from build123d import *

# Parameters (mm, degrees)
SKETCH1_R           = 3.2639
BOSS_EXTRUDE1_DEPTH = 1.5875
SKETCH2_R           = 12.7
CUT_EXTRUDE1_DEPTH  = 27.658658303


with BuildPart() as part:
    # Sketch1 → Boss-Extrude1 (new body)
    with BuildSketch(Plane(origin=(0, 0, 0), x_dir=(1, 0, 0), z_dir=(0, 1, 0))):
        with BuildLine():
            Line((-25.4, 7.9375), (0, 7.9375))
            ThreePointArc((0, 7.9375), (7.9375, 0), (0, -7.9375))
            Line((0, -7.9375), (-25.4, -7.9375))
            Line((-25.4, -7.9375), (-25.4, 7.9375))
        make_face()
        with Locations(Location((0, 0, 0), (0, 0, 270))):
            Circle(SKETCH1_R, mode=Mode.SUBTRACT)
    extrude(amount=BOSS_EXTRUDE1_DEPTH)

    # Sketch2 → Cut-Extrude1 (cut, through all)
    with BuildSketch(Plane(origin=(0, 1.5875, 0), x_dir=(1, 0, 0), z_dir=(0, 1, 0))):
        with Locations((-25.4, 0)):
            Circle(SKETCH2_R)
    extrude(amount=-CUT_EXTRUDE1_DEPTH, mode=Mode.SUBTRACT)


solid = part.part
Part model, mm, in its own coordinate system. Round coordinates to 2 decimals unless told otherwise and drop trailing zeros. Order: outer loops, then holes, each group sorted by start corner. A loop starts at its lowest first (then second) coordinate and runs counter-clockwise, first axis right, second up. Notation, with made-up numbers: (-1, 67) -> (39, 67) arc R7 ccw to (39, 80) -> close; hole circle Ø9 at (-25.75, 55). An arc over 180 degrees is marked (long way). Put each result on its own line as item: value.
Q1. Band-saw the part on D-D (x = 6.25). Give the cut face in (y, z), and give its area (3 significant figures).
From the geometry:
outline: (0, -4.89) -> (1.59, -4.89) -> (1.59, 4.89) -> (0, 4.89) -> close
area: 15.5 mm2
Q2. Band-saw the part on B-B (x = 2.25). Give the cut face in (y, z).
From the geometry:
outline: (0, -7.61) -> (1.59, -7.61) -> (1.59, -2.36) -> (0, -2.36) -> close; (0, 2.36) -> (1.59, 2.36) -> (1.59, 7.61) -> (0, 7.61) -> close
Q3. Band-saw the part on C-C (y = 1.3). Give the cut face in (x, z) (1 decimal), and give its area (3 significant figures).
From the geometry:
outline: (-15.5, -7.9) -> (0, -7.9) arc R7.9 ccw to (0, 7.9) -> (-15.5, 7.9) arc R12.7 cw to start; hole circle Ø6.5 at (0, 0)
area: 281 mm2
Q4. Pull direction Z, two halves, no side cores. Call faces 1 (the face through (7.936, 0.783, -0.175)), 2 (the face through (-4, 1.588, 0)), 3 (the face through (-8, 1, 7.938)), 4 (the face through (-3.186, 0.783, -0.708)): pulls with the +Z half, pulls with the -Z half, needs draft (parallel to the pull), parting line crosses it, or undercut.
From the geometry:
face 1: parting line crosses it
face 2: needs draft
face 3: pulls with the +Z half
face 4: undercut
Q5. Band-saw the part on A-A (z = 0). Give the cut face in (x, y), and give its area (3 significant figures).
From the geometry:
outline: (-12.7, 0) -> (-3.26, 0) -> (-3.26, 1.59) -> (-12.7, 1.59) -> close; (3.26, 0) -> (7.94, 0) -> (7.94, 1.59) -> (3.26, 1.59) -> close
area: 22.4 mm2
Q6. Wall check: line 1 (Z direction, x = -3, y = 1.25); line 2 (Z direction, x = -0.5, y = 1.1); line 3 (X direction, y = 0.2, z = 2.75). Give the ranges that are in metal, low to high. Write a range as [from, to].
From the geometry:
line 1: z = [-7.94, -1.29], [1.29, 7.94]
line 2: z = [-7.94, -3.23], [3.23, 7.94]
line 3: x = [-13, -1.76], [1.76, 7.45]
